Autodesk Inventor part; units mm, degrees
ref_plane "YZ Plane" through (0, 0, 0) normal (1, 0, 0) x (0, 1, 0)
ref_plane "XZ Plane" through (0, 0, 0) normal (0, 1, 0) x (-1, 0, 0)
ref_plane "XY Plane" through (0, 0, 0) normal (0, 0, 1) x (1, 0, 0)
sketch "Esquisse1" plane through (0, 0, 0) normal (0, 0, 1) x (1, 0, 0)
  circle A0 centre (0, 0) radius 10
  circle A1 centre (0, 0) radius 5
  dimension "d0" = 20
  dimension "d1" = 10
extrude "Extrusion1" add sketch "Esquisse1" along normal blind 120
sketch "Esquisse2" plane through (0, 0, 0) normal (0, 1, 0) x (-1, 0, 0)
  line L0 (0, 0) -> (0, 5)
  line L1 (10, 120) -> (-10, 120)
  line L2 (0, 120) -> (0, 115)
  dimension "d4" = 5
  dimension "d5" = 5
hole "Perçage1" at (0, 0, 5) at (0, 0, 115) direction (0, -1, 0) diameter 4 end through all both
properties part number "tubelong_rocker"
Geometry: final body of the model. Coordinates: model frame, mm. Coordinates: 2 decimals unless noted, no trailing zeros. Order: outer loops, then holes, each group sorted by start corner. A loop starts at its lowest first (then second) coordinate and runs counter-clockwise, first axis right, second up. Notation, with made-up numbers: (-27.75, -22) -> (-13.75, -22) arc R17 ccw to (-13.75, 11) -> close; hole circle Ø11 at (88, 72). An arc over 180 degrees is marked (long way). Answer in a Markdown table with one row per item.
Item 1: Section C-C on z = 115. Output: boundary loops of the cut face in (x, y), plus the area to 3 significant figures.
Return value:
| item | result |
|---|---|
| outline | (-2, -9.8) -> (-2, -4.58) arc R5 cw to (-2, 4.58) -> (-2, 9.8) arc R10 ccw to start; (2, -9.8) arc R10 ccw to (2, 9.8) -> (2, 4.58) arc R5 cw to (2, -4.58) -> close |
| area | 195 mm² |
Item 2: Section D-D on y = -7. Output: boundary loops of the cut face in (x, z).
Return value:
| item | result |
|---|---|
| outline | (-7.14, 0) -> (7.14, 0) -> (7.14, 120) -> (-7.14, 120) -> close; hole circle Ø4 at (0, 5); hole circle Ø4 at (0, 115) |
Item 3: Section B-B on x = 0. Output: boundary loops of the cut face in (y, z).
Return value:
| item | result |
|---|---|
| outline | (-10, 0) -> (-5, 0) -> (-5, 3) -> (-10, 3) -> close; (-10, 7) -> (-5, 7) -> (-5, 113) -> (-10, 113) -> close; (-10, 117) -> (-5, 117) -> (-5, 120) -> (-10, 120) -> close; (5, 0) -> (10, 0) -> (10, 3) -> (5, 3) -> close; (5, 7) -> (10, 7) -> (10, 113) -> (5, 113) -> close; (5, 117) -> (10, 117) -> (10, 120) -> (5, 120) -> close |
Item 4: Draft query along Z for faces 1 (the flat face through (2, 5, 0)), 2 (the cylindrical face through (0, -7, 113)), 3 (the flat face through (2, 5, 120)). Return one class per face: released by +Z, released by -Z, zero draft, split by the parting line, or undercut.
Return value:
| item | result |
|---|---|
| face 1 | released by -Z |
| face 2 | undercut |
| face 3 | released by +Z |
Item 5: Section A-A on y = 0. Output: boundary loops of the cut face in (x, z).
Return value:
| item | result |
|---|---|
| outline | (-10, 0) -> (-5, 0) -> (-5, 120) -> (-10, 120) -> close; (5, 0) -> (10, 0) -> (10, 120) -> (5, 120) -> close |
Item 6: Ray query, L1, parallel to Z at x = 0, y = 8.1; L2, parallel to Z at x = 0.5, y = 8.5; L3, parallel to Y at x = 0, z = 106. Return the intervals inside material, ascending.
Return value:
| item | result |
|---|---|
| L1 | z = 0 to 3, 7 to 113, 117 to 120 |
| L2 | z = 0 to 3.06, 6.94 to 113.06, 116.94 to 120 |
| L3 | y = -10 to -5, 5 to 10 |
Item 7: Contact query for flat-ended pins moving along their axis: P1, Ø2.5, axis at x = 0, z = 115, coming from the +Y side; P2, Ø6, axis at y = 8, z = 35, coming from the +X side; P3, Ø5, axis at y = 5, z = 56, coming from the -X side; P4, Ø1, axis at x = -6, z = 61.5, coming from the +Y side. Output: stop coordinate, or through.
Return value:
| item | result |
|---|---|
| P1 | passes through |
| P2 | stops at x = 8.66 |
| P3 | stops at x = -9.68 |
| P4 | stops at y = 8.35 |
